Input: dimensioned drawing with shaded views. Units: mm. Origin: part minimum x, y, z. A direction names the side the tool comes from. Coordinates: 2 decimals unless noted, no trailing zeros. Write each loop counter-clockwise with the first axis right and the second up, starting at its lowest first coordinate (ties: lowest second). Pieces come first, ordered by that corner, then holes. Notation, with made-up numbers: (-33, 60) -> (-8, 60) arc R17 cw to (-8, 93) -> close; hole circle Ø11 at (72.25, 22.5). An arc over 180 degrees is marked (long way). One line per item, written item: value. Start each with the question number.
1. Section query C-C, the plane y = 4. Output: boundary loops of the cut face in (x, z).
2. Access query for the marked faces 1 and 2. Directions: +Z, -Z, +X, -X, +Y, -Y. A direction counts if a zero-diameter tool reaches every point of the face in a straight line with its end or side. Return the directions, or none.
3. Section query B-B, the plane z = 4. Output: boundary loops of the cut face in (x, y), and give its area (3 significant figures).
4. First-contact query: P1, Ø1, axis at y = 33, z = 5.5, coming from the +X side; P2, Ø0.5, axis at y = 0.5, z = 5.5, coming from the +X side; P3, Ø0.8, axis at y = 0.5, z = 6.5, coming from the -X side (1 decimal). Flat tips, straight axial feed; report the tip coordinate or a pass-through.
5. Section query A-A, the plane x = 4. Output: boundary loops of the cut face in (y, z), and give its area (3 significant figures).
6. Line query: line 1 (Y direction, x = 4.75, z = 7.5); line 2 (Y direction, x = 1, z = 3.75); line 3 (X direction, y = 33.5, z = 5.5). Output: solid intervals per line, ascending.
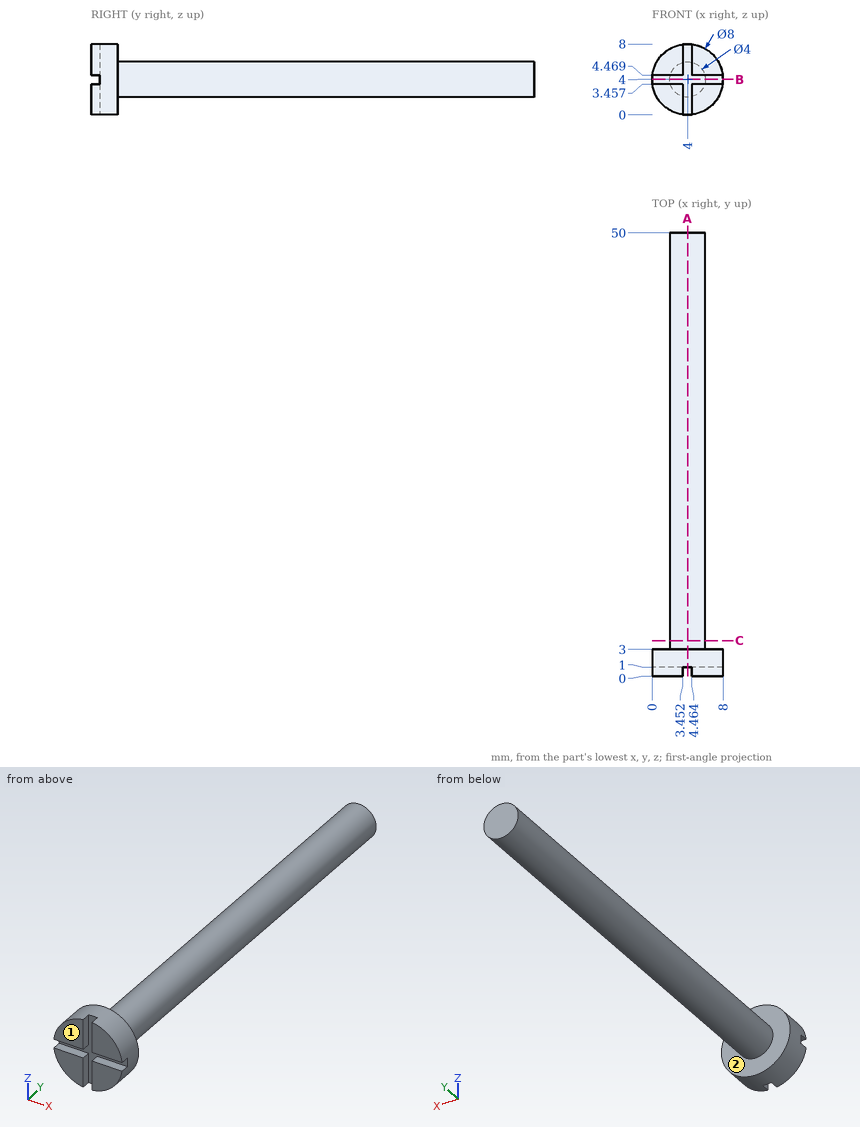
Computed values:
1. outline: circle Ø4 at (4, 4)
2. face 1: +Z, -Z, +X, -X, -Y
2. face 2: +Y
3. outline: (0, 1) -> (8, 1) -> (8, 3) -> (6, 3) -> (6, 50) -> (2, 50) -> (2, 3) -> (0, 3) -> close
3. area: 204 mm²
4. P1: stops at x = 5.73
4. P2: stops at x = 7.8
4. P3: stops at x = 0.6
5. outline: (1, 0) -> (3, 0) -> (3, 2) -> (50, 2) -> (50, 6) -> (3, 6) -> (3, 8) -> (1, 8) -> close
5. area: 204 mm²
6. line 1: y = 0 to 3
6. line 2: y = 1 to 3
6. line 3: x = 2.68 to 5.32
